Model file for the job. Use its own axes, mm. Face numbers are marked on the shaded views. Round coordinates to 2 decimals unless told otherwise and drop trailing zeros. Order: outer loops, then holes, each group sorted by start corner. A loop starts at its lowest first (then second) coordinate and runs counter-clockwise, first axis right, second up. Notation, with made-up numbers: (55.5, 82.5) -> (99.5, 82.5) arc R29 cw to (99.5, 104.5) -> close; hole circle Ø6 at (-17.75, 48). An arc over 180 degrees is marked (long way). Use CSV: the item, a comma, the result in double quotes.
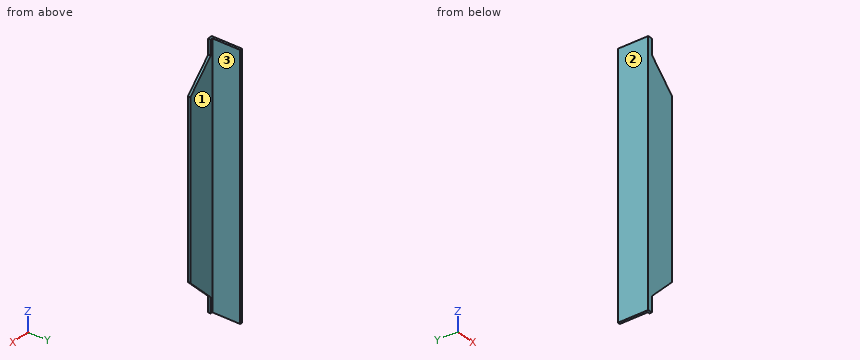
```python
from build123d import *

# Parameters (mm, degrees)
SKETCH_1_W          = 100
SKETCH_1_H          = 100
EXTRUDE_1_DEPTH     = 840
SKETCH_2_W          = 92
SKETCH_2_H          = 92
CUT_EXTRUDE_1_DEPTH = 852.821577562
CUT_EXTRUDE_3_DEPTH = 851.919502656


with BuildPart() as part:
    # 草图1 → 凸台-拉伸1 (new body)
    with BuildSketch(Plane.XY):
        with Locations((50, 50)):
            Rectangle(SKETCH_1_W, SKETCH_1_H)
    extrude(amount=EXTRUDE_1_DEPTH)

    # 草图2 → 切除-拉伸1 (cut, through all)
    with BuildSketch(Plane.XY.offset(840)):
        with Locations((54, 54)):
            Rectangle(SKETCH_2_W, SKETCH_2_H)
    extrude(amount=-CUT_EXTRUDE_1_DEPTH, mode=Mode.SUBTRACT)

    # 草图4 → 切除-拉伸3 (cut, through all)
    with BuildSketch(Plane(origin=(0, 8, 0), x_dir=(1, 0, 0), z_dir=(0, 1, 0))):
        Polygon((15, 0), (15, -50), (100, -135), (100, 0), align=None)
        Polygon((15, -840), (15, -790), (100, -705), (100, -840), align=None)
    extrude(amount=-CUT_EXTRUDE_3_DEPTH, mode=Mode.SUBTRACT)


solid = part.part
```
Q1. Probe line 1 along Y through (x, z) = (42, 91.5). List the from-to ranges inside material, lowest first.
From the geometry:
line 1,"y = 0 to 8"
Q2. Cut at C-C (y = 77). Give the cut face in (x, z).
From the geometry:
outline,"(0, 0) -> (8, 0) -> (8, 840) -> (0, 840) -> close"
Q3. Mould opens along X. For the marked faces 1, 2 and 3 say: +X half, -X half, draft (parallel to the pull), parting line (faces both ways), or undercut.
From the geometry:
face 1,"draft"
face 2,"-X half"
face 3,"+X half"
Q4. Cut at B-B (z = 748). Give the cut face in (x, y).
From the geometry:
outline,"(0, 0) -> (57, 0) -> (57, 8) -> (8, 8) -> (8, 100) -> (0, 100) -> close"
Q5. Cut at A-A (x = 36.5). Give the cut face in (y, z).
From the geometry:
outline,"(0, 71.5) -> (8, 71.5) -> (8, 768.5) -> (0, 768.5) -> close"
Q6. Pin check, flat tips, straight feed: pin 1 (6 mm diameter, centred on y = 82, z = 724.5, fed in from +X); pin 2 (2.5 mm diameter, centred on y = 5, z = 804.5, fed in from +X). Stop position of each tip, or through.
From the geometry:
pin 1,"stops at x = 8"
pin 2,"stops at x = 15"
Q7. Cut at D-D (z = 77.5). Give the cut face in (x, y), plus the area to 3 significant figures.
From the geometry:
outline,"(0, 0) -> (42.5, 0) -> (42.5, 8) -> (8, 8) -> (8, 100) -> (0, 100) -> close"
area,"1,080 mm²"
